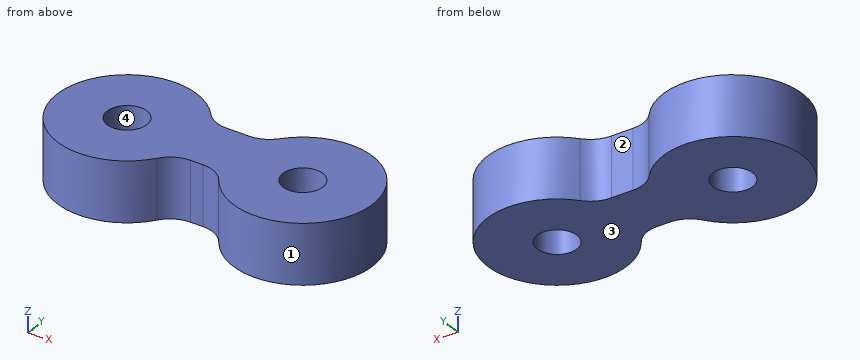
```python
from build123d import *

# Parameters (mm, degrees)
SKETCH_1_R      = 1
EXTRUDE_1_DEPTH = 3
FILLET_1_R      = 1.524


with BuildPart() as part:
    # 스케치1 → 보스-돌출1 (new body)
    with BuildSketch(Plane.XY):
        with BuildLine():
            ThreePointArc((1.360201973, -0.016393318), (7.940776925, -1.84176367), (1.212873871, -3.012773539))
            ThreePointArc((1.212873871, -3.012773539), (0, -2.999007865), (-1.212873871, -3.012773539))
            ThreePointArc((-1.212873871, -3.012773539), (-7.940776925, -1.84176367), (-1.360201973, -0.016393318))
            ThreePointArc((-1.360201973, -0.016393318), (0, 0), (1.360201973, -0.016393318))
        make_face()
        with Locations((-4.445, -1.669880884)):
            Circle(SKETCH_1_R, mode=Mode.SUBTRACT)
        with Locations((4.445, -1.669880884)):
            Circle(SKETCH_1_R, mode=Mode.SUBTRACT)
    extrude(amount=EXTRUDE_1_DEPTH)

    # 필렛1
    fillet_1_edges = [part.edges().sort_by_distance(p)[0] for p in [
        (-1.360201973, -0.016393318, 1.5),
        (1.360201973, -0.016393318, 1.5),
        (1.212873871, -3.012773539, 1.5),
        (-1.212873871, -3.012773539, 1.5),
    ]]
    fillet(fillet_1_edges, radius=FILLET_1_R)


solid = part.part
```
CAD build for the part. Positions are in the model's coordinates, mm. Face numbers are marked on the shaded views. A direction names the side the tool comes from. Round coordinates to 2 decimals unless told otherwise and drop trailing zeros. Write each loop counter-clockwise with the first axis right and the second up, starting at its lowest first coordinate (ties: lowest second). Pieces come first, ordered by that corner, then holes. Notation, with made-up numbers: (68.5, 75.5) - (114.5, 75.5) arc R26 cw to (114.5, 104.5) - close; hole circle Ø4 at (52, 11). An arc over 180 degrees is marked (long way). Return JSON: item names as keys, results as strings. Group by question number.
Item 1: Flat gauge pins, fed straight in: pin 1 Ø1.5 at (x, z) = (2, 1.5) entering from +Y; pin 2 Ø1 at (x, y) = (1, 1) entering from -Z. Where does each tip first touch, or does it go through?
Item 2: Band-saw the part on C-C on z = 1.05. State how many separate pieces and enclosed holes the cut face has, plus the area to 3 significant figures.
Item 3: Mould opens along X. For the marked faces 3 and 4 say: +X half, -X half, draft (parallel to the pull), parting line (faces both ways), or undercut.
Item 4: Band-saw the part on B-B on x = 4.25. List the corners of the cut face in (y, z), plus the area to 3 significant figures.
Item 5: Probe probe 1 along Y at (x, z) = (4.5, 2.45); probe 2 along X at (y, z) = (-1.25, 2.15); probe 3 along X at (y, z) = (-2.25, 0.75). List the from-to ranges inside material, lowest first.
Item 6: Band-saw the part on D-D on x = 2.25. List the corners of the cut face in (y, z), plus the area to 3 significant figures.
Item 7: 3-axis set-ups, long thin cutter, end or side, ignore diameter. For the marked faces 1 and 2: which of +Z, -Z, +X, -X, +Y, -Y reach the whole face in a straight line?
Item 8: Band-saw the part on A-A on y = 0.75. List the corners of the cut face in (x, z).
Resolved:
{
 "1": {"pin 1": "stops at y = 1.39", "pin 2": "passes through"},
 "2": {"separate pieces": "1", "enclosed holes": "2", "area": "77.5 mm²"},
 "3": {"face 3": "draft", "face 4": "undercut"},
 "4": {"outline": "(-5.16, 0) - (-2.65, 0) - (-2.65, 3) - (-5.16, 3) - close; (-0.69, 0) - (1.82, 0) - (1.82, 3) - (-0.69, 3) - close", "area": "15.1 mm²"},
 "5": {"probe 1": "y = -5.17 to -2.67, -0.67 to 1.83", "probe 2": "x = -7.92 to -5.35, -3.54 to 3.54, 5.35 to 7.92", "probe 3": "x = -7.9 to -5.26, -3.63 to 3.63, 5.26 to 7.9"},
 "6": {"outline": "(-4.4, 0) - (1.06, 0) - (1.06, 3) - (-4.4, 3) - close", "area": "16.4 mm²"},
 "7": {"face 1": "+Z, -Z", "face 2": "+Z, -Z, +Y"},
 "8": {"outline": "(-6.97, 0) - (-1.92, 0) - (-1.92, 3) - (-6.97, 3) - close; (1.92, 0) - (6.97, 0) - (6.97, 3) - (1.92, 3) - close"}
}
